Design review of the part shown in the three views and the two pictorial views. Dimensions are in mm from the part's minimum x, y and z. Coordinates: 2 decimals unless noted, no trailing zeros. Write each loop counter-clockwise with the first axis right and the second up, starting at its lowest first coordinate (ties: lowest second). Pieces come first, ordered by that corner, then holes. Notation, with made-up numbers: (69, 50) -> (76, 50) arc R36 cw to (76, 87) -> close; hole circle Ø6 at (18.25, 5.5). An arc over 180 degrees is marked (long way). Write each question's results on one line, items separated by ' | '.
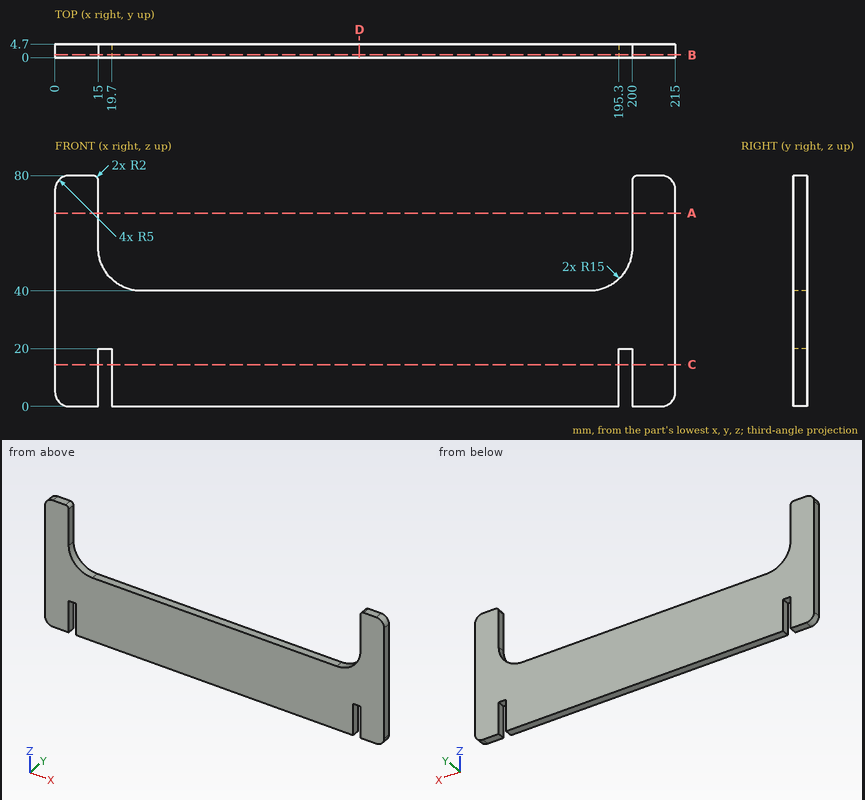
Q1. Add section B-B (y = 0.9). Write out the cut boundary in (x, z).
Solution:
outline: (0, 5) arc R5 ccw to (5, 0) -> (15, 0) -> (15, 20) -> (19.7, 20) -> (19.7, 0) -> (195.3, 0) -> (195.3, 20) -> (200, 20) -> (200, 0) -> (210, 0) arc R5 ccw to (215, 5) -> (215, 75) arc R5 ccw to (210, 80) -> (202, 80) arc R2 ccw to (200, 78) -> (200, 55) arc R15 cw to (185, 40) -> (30, 40) arc R15 cw to (15, 55) -> (15, 78) arc R2 ccw to (13, 80) -> (5, 80) arc R5 ccw to (0, 75) -> close
Q2. For line 1 (X direction, y = 1, z = 15); line 2 (X direction, y = 2.35, z = 60.5); line 3 (X direction, y = 1.05, z = 43), list the stretches that pass through material, from the lowest coordinate up. Write a range as from..to.
Solution:
line 1: 0..15, 19.7..195.3, 200..215 | line 2: 0..15, 200..215 | line 3: 0..21, 194..215
Q3. Add section C-C (z = 14.5). Write out the cut boundary in (x, y), plus the area to 3 significant figures.
Solution:
outline: (0, 0) -> (15, 0) -> (15, 4.7) -> (0, 4.7) -> close; (19.7, 0) -> (195.3, 0) -> (195.3, 4.7) -> (19.7, 4.7) -> close; (200, 0) -> (215, 0) -> (215, 4.7) -> (200, 4.7) -> close | area: 966 mm²
Q4. Clearance check with flat-ended pins moving along their axes: P1, Ø10, axis at x = 152, z = 49, coming from the -Y side; P2, Ø2.5, axis at x = 124, y = 1.5, coming from the +Z side. State where each tip first meets the part, or that it passes through.
Solution:
P1: through | P2: z = 40
Q5. Add section D-D (x = 105.5). Write out the cut boundary in (y, z), plus the area to 3 significant figures.
Solution:
outline: (0, 0) -> (4.7, 0) -> (4.7, 40) -> (0, 40) -> close | area: 188 mm²
Q6. Add section A-A (z = 67). Write out the cut boundary in (x, y).
Solution:
outline: (0, 0) -> (15, 0) -> (15, 4.7) -> (0, 4.7) -> close; (200, 0) -> (215, 0) -> (215, 4.7) -> (200, 4.7) -> close
